Design review of the part built by this model. Coordinates are the model's own, in mm. Round coordinates to 2 decimals unless told otherwise and drop trailing zeros. Order: outer loops, then holes, each group sorted by start corner. A loop starts at its lowest first (then second) coordinate and runs counter-clockwise, first axis right, second up. Notation, with made-up numbers: M 41.25,24.25 L 89.25,24.25 A12 cw 89.25,36.25 Z; hole C 59,61.5 d6. An arc over 180 degrees is marked long. Write each question's results on one line, items separated by ' | '. Start each with the question number.
Item 1: Take a section at A-A, the plane y = 60.5. Write out the cut boundary in (x, z).
Item 2: The part is to be moulded in two halves that separate along Y. For faces 1 (the flat face through (69.52, 30.17, 2.64)), 2 (the cylindrical face through (-0.43, -82.04, 2.57)), 3 (the flat face through (70.324, 27.755, 2.64)), 4 (the flat face through (-67, 19, 0)), say which applies: +Y half, -Y half, draft (parallel to the pull), parting line (faces both ways), or undercut.
Item 3: Wall thickness on line 1 (Y direction, x = 52.5, z = 2.55); line 2 (Y direction, x = 53, z = 1.3) (3 decimals); line 3 (X direction, y = 53.5, z = 4.95): over which ranges is each line inside the solid? List them lowest first. Write a range as [from, to].
Item 4: Clearance check with flat-ended pins moving along their axes: pin 1 (1.6 mm diameter, centred on x = 75.692, y = 0, fed in from +Z); pin 2 (3 mm diameter, centred on y = 28.5, z = 2, fed in from -X). State where each tip first meets the part, or that it passes through.
Item 5: Take a section at C-C, the plane z = 1.6. Count the separate pieces of the cut face and the enclosed holes in it, plus the area to 3 significant figures.
Item 6: Take a section at B-B, the plane x = -49. Write out the cut boundary in (y, z), plus the area to 3 significant figures.
```python
from build123d import *

# Parameters (mm, degrees)
SKETCH4_R             = 82.042
BOSS_EXTRUDE2_DEPTH   = 5.207
SKETCH5_R             = 69.342
CUT_EXTRUDE5_DEPTH    = 6.207
CUT_EXTRUDE11_DEPTH   = 6.207
F_6_32_TAPPED_HOLE1_D = 2.7051


with BuildPart() as part:
    # Sketch4 → Boss-Extrude2 (new body)
    with BuildSketch(Plane.XY):
        Circle(SKETCH4_R)
    extrude(amount=BOSS_EXTRUDE2_DEPTH)

    # Sketch5 → Cut-Extrude5 (cut, through all)
    with BuildSketch(Plane.XY.offset(5.207)):
        Circle(SKETCH5_R)
    extrude(amount=-CUT_EXTRUDE5_DEPTH, mode=Mode.SUBTRACT)

    # Sketch8 → Cut-Extrude11 (cut, through all)
    with BuildSketch(Plane.XY.offset(5.207)):
        Polygon((81.764215182, 35.242484939), (62.990983081, 27.466357594), (63.962998999, 25.119703581), (82.7362311, 32.895830927), align=None)
        Polygon((32.812445144, 75.89758015), (30.465791131, 76.869596069), (29.979783172, 75.696269062), (32.326437185, 74.724253144), align=None)
        Polygon((-30.465791131, 76.869596069), (-32.812445144, 75.89758015), (-32.326437185, 74.724253144), (-29.979783172, 75.696269062), align=None)
        Polygon((-75.89758015, 32.812445144), (-76.869596069, 30.465791131), (-75.696269062, 29.979783172), (-74.724253144, 32.326437185), align=None)
        Polygon((-76.869596069, -30.465791131), (-75.89758015, -32.812445144), (-74.724253144, -32.326437185), (-75.696269062, -29.979783172), align=None)
        Polygon((-32.812445144, -75.89758015), (-30.465791131, -76.869596069), (-29.979783172, -75.696269062), (-32.326437185, -74.724253144), align=None)
        Polygon((30.465791131, -76.869596069), (32.812445144, -75.89758015), (32.326437185, -74.724253144), (29.979783172, -75.696269062), align=None)
        Polygon((75.89758015, -32.812445144), (76.869596069, -30.465791131), (75.696269062, -29.979783172), (74.724253144, -32.326437185), align=None)
    extrude(amount=-CUT_EXTRUDE11_DEPTH, mode=Mode.SUBTRACT)

    # #6-32 Tapped Hole1 (through all)
    with Locations(Plane.XY.offset(5.207)):
        with Locations((75.692, 0), (53.522326482, -53.522326482), (0, -75.692), (-53.522326482, -53.522326482), (-75.692, 0), (-53.522326482, 53.522326482), (0, 75.692), (53.522326482, 53.522326482)):
            Hole(F_6_32_TAPPED_HOLE1_D / 2)


solid = part.part
```
Results list:
1) outline: M -55.41,0 L -33.88,0 L -33.88,5.21 L -55.41,5.21 Z; M 33.88,0 L 55.41,0 L 55.41,5.21 L 33.88,5.21 Z
2) face 1: undercut | face 2: -Y half | face 3: undercut | face 4: draft
3) line 1: [-63.04, -54.41], [-52.64, -45.3], [45.3, 52.64], [54.41, 63.04] | line 2: [-62.625, -54.77], [-52.275, -44.714], [44.714, 52.275], [54.77, 62.625] | line 3: [-62.2, -54.87], [-52.17, -44.11], [44.11, 52.17], [54.87, 62.2]
4) pin 1: through | pin 2: x = -77.47
5) separate pieces: 1 | enclosed holes: 8 | area: 5,950 mm²
6) outline: M -65.8,0 L -49.06,0 L -49.06,5.21 L -65.8,5.21 Z; M 49.06,0 L 65.8,0 L 65.8,5.21 L 49.06,5.21 Z | area: 174 mm²
